```python
from build123d import *

# Parameters (mm, degrees)
SKETCH1_R           = 11.5
SKETCH1_R_2         = 1.25
SKETCH1_R_3         = 1.5
BOSS_EXTRUDE1_DEPTH = 2
SKETCH2_R           = 4.5
SKETCH2_R_2         = 1.5
BOSS_EXTRUDE2_DEPTH = 2.5
SKETCH3_R           = 2.25
CUT_EXTRUDE1_DEPTH  = 3.6


with BuildPart() as part:
    # Sketch1 → Boss-Extrude1 (new body)
    with BuildSketch(Plane(origin=(0, 0, 0), x_dir=(1, 0, 0), z_dir=(0, 1, 0))):
        with Locations(Location((0, 0, 0), (0, 0, 270))):
            Circle(SKETCH1_R)
        with Locations(Location((-4.949747468, 4.949747468, 0), (0, 0, 270))):
            Circle(SKETCH1_R_2, mode=Mode.SUBTRACT)
        with Locations(Location((4.949747468, 4.949747468, 0), (0, 0, 270))):
            Circle(SKETCH1_R_2, mode=Mode.SUBTRACT)
        with Locations(Location((4.949747468, -4.949747468, 0), (0, 0, 270))):
            Circle(SKETCH1_R_2, mode=Mode.SUBTRACT)
        with Locations(Location((-4.949747468, -4.949747468, 0), (0, 0, 270))):
            Circle(SKETCH1_R_2, mode=Mode.SUBTRACT)
        with Locations(Location((0, 0, 0), (0, 0, 270))):
            Circle(SKETCH1_R_3, mode=Mode.SUBTRACT)
    extrude(amount=BOSS_EXTRUDE1_DEPTH)

    # Sketch2 → Boss-Extrude2 (add)
    with BuildSketch(Plane(origin=(0, 2, 0), x_dir=(1, 0, 0), z_dir=(0, 1, 0))):
        with Locations(Location((0, 0, 0), (0, 0, 270))):
            Circle(SKETCH2_R)
        with Locations(Location((0, 0, 0), (0, 0, 270))):
            Circle(SKETCH2_R_2, mode=Mode.SUBTRACT)
    extrude(amount=BOSS_EXTRUDE2_DEPTH)

    # Sketch3 → Cut-Extrude1 (cut)
    with BuildSketch(Plane(origin=(0, 4.5, 0), x_dir=(1, 0, 0), z_dir=(0, 1, 0))):
        with Locations(Location((0, 0, 0), (0, 0, 270))):
            Circle(SKETCH3_R)
    extrude(amount=-CUT_EXTRUDE1_DEPTH, mode=Mode.SUBTRACT)


solid = part.part
```
Geometry check sheet. Reference: the model listing, model coordinates, mm. A direction names the side the tool comes from. Coordinates: 2 decimals unless noted, no trailing zeros. Write each loop counter-clockwise with the first axis right and the second up, starting at its lowest first coordinate (ties: lowest second). Pieces come first, ordered by that corner, then holes. Notation, with made-up numbers: M 56.5,-9.75 L 96.5,-9.75 A20 cw 96.5,25.25 Z; hole C 11,5 d10. An arc over 180 degrees is marked long. One line per item, written item: value. Start each with the question number.
(1) Sectioned sample at A-A, the plane z = 0. Enter the section's corners in (x, y).
(2) Sectioned sample at C-C, the plane x = 4. Enter the section's corners in (y, z), and give its area (3 significant figures).
(3) Scan lines: line 1 along X through (y, z) = (0.8, 4); line 2 along X through (y, z) = (1.65, 0); line 3 along X through (y, z) = (1.6, 4.5). Record each from-to range of solid material in increasing order. Write a range as [from, to].
(4) Tool access check on faces 4 (the face through (0, 0.9, -2)), 5 (the face through (-6.17, 0.99, -5.22)). Record the directions out of +Z, -Z, +X, -X, +Y, -Y that give a thin tool (end or side, any length) a straight path to the whole face; none if there is none.
(5) Release check for a two-part mould opening along X. For faces 1 (the face through (1.352, 3.232, 4.292)), 2 (the face through (-2, 4.5, 2)), 3 (the face through (-6.17, 0.99, 4.68)) record: released by +X, released by -X, zero draft, split by the parting line, or undercut.
(6) Depth check by flat-ended pin: pin 1 (2 mm diameter, centred on x = -4.95, z = 4.95, fed in from +Y); pin 2 (1.5 mm diameter, centred on x = -6.5, y = 0.5, fed in from +Z); pin 3 (2 mm diameter, centred on y = 2.5, z = -8, fed in from -X); pin 4 (4 mm diameter, centred on x = -4.95, z = -4.95, fed in from +Y). Enter the tip coordinate at first touch or a pass-through.
(7) Sectioned sample at B-B, the plane x = 0. Enter the section's corners in (y, z).
(8) Sectioned sample at D-D, the plane y = 3.45. Enter the section's corners in (x, z), and give its area (3 significant figures).
Filled sheet:
1. outline: M -11.5,0 L -1.5,0 L -1.5,0.9 L -2.25,0.9 L -2.25,4.5 L -4.5,4.5 L -4.5,2 L -11.5,2 Z; M 1.5,0 L 11.5,0 L 11.5,2 L 4.5,2 L 4.5,4.5 L 2.25,4.5 L 2.25,0.9 L 1.5,0.9 Z
2. outline: M 0,-10.78 L 2,-10.78 L 2,-5.76 L 0,-5.76 Z; M 0,-4.14 L 2,-4.14 L 2,-2.06 L 4.5,-2.06 L 4.5,2.06 L 2,2.06 L 2,4.14 L 0,4.14 Z; M 0,5.76 L 2,5.76 L 2,10.78 L 0,10.78 Z
2. area: 46.9 mm²
3. line 1: [-10.78, -5.76], [-4.14, 4.14], [5.76, 10.78]
3. line 2: [-11.5, -2.25], [2.25, 11.5]
3. line 3: [-10.58, -6.12], [-3.78, 3.78], [6.12, 10.58]
4. face 4: +Y
4. face 5: +Y, -Y
5. face 1: split by the parting line
5. face 2: zero draft
5. face 3: undercut
6. pin 1: through
6. pin 2: z = 9.96
6. pin 3: x = -9.02
6. pin 4: y = 2
7. outline: M 0,-11.5 L 2,-11.5 L 2,-4.5 L 4.5,-4.5 L 4.5,-2.25 L 0.9,-2.25 L 0.9,-1.5 L 0,-1.5 Z; M 0,1.5 L 0.9,1.5 L 0.9,2.25 L 4.5,2.25 L 4.5,4.5 L 2,4.5 L 2,11.5 L 0,11.5 Z
8. outline: C 0,0 d9; hole C 0,0 d4.5
8. area: 47.7 mm²
